Model file for the job. Use its own axes, mm. Face numbers are marked on the shaded views. A direction names the side the tool comes from. Round coordinates to 2 decimals unless told otherwise and drop trailing zeros. Loops run counter-clockwise (first coordinate to the right, second up) from the corner with the lowest first, then second, coordinate; pieces in that order, holes last.
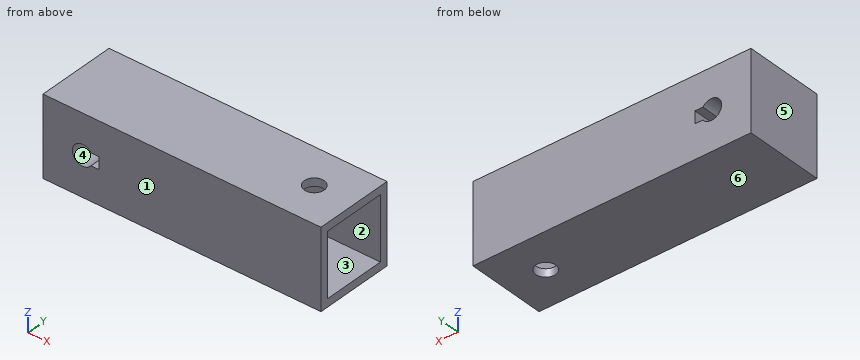
from build123d import *

# Parameters (mm, degrees)
SKETCH2_W               = 140
SKETCH2_H               = 40
SKETCH2_R               = 5.2
BOSS_EXTRUDE1_DEPTH     = 40
CUT_EXTRUDE1_DEPTH      = 84.066238629
CUT_EXTRUDE1_DEPTH_BACK = 84.066238629
SKETCH3_R               = 5
CUT_EXTRUDE5_DEPTH      = 84.066238629
CUT_EXTRUDE5_DEPTH_BACK = 84.066238629
SKETCH7_W               = 2
SKETCH7_H               = 6.131883886
CUT_EXTRUDE6_START      = 70
SKETCH8_W               = 32
SKETCH8_H               = 32
CUT_EXTRUDE6_DEPTH      = 80


with BuildPart() as part:
    # Sketch2 → Boss-Extrude1 (new body)
    with BuildSketch(Plane(origin=(0, 0, 0), x_dir=(1, 0, 0), z_dir=(0, 1, 0))):
        Rectangle(SKETCH2_W, SKETCH2_H)
        with Locations(Location((-50, 0, 0), (0, 0, 270))):
            Circle(SKETCH2_R, mode=Mode.SUBTRACT)
    extrude(amount=BOSS_EXTRUDE1_DEPTH)

    # Sketch3 → Cut-Extrude1 (cut, two sides: drawn at the far end of the back side and taken through both)
    with BuildSketch(Plane.XY.offset(-CUT_EXTRUDE1_DEPTH_BACK)):
        with Locations((50, 20)):
            Circle(SKETCH3_R)
    extrude(amount=CUT_EXTRUDE1_DEPTH + CUT_EXTRUDE1_DEPTH_BACK, mode=Mode.SUBTRACT)

    # Sketch7 → Cut-Extrude5 (cut, two sides: drawn at the far end of the back side and taken through both)
    with BuildSketch(Plane(origin=(0, 0, 0), x_dir=(1, 0, 0), z_dir=(0, 1, 0)).offset(-CUT_EXTRUDE5_DEPTH_BACK)):
        with Locations((-42.8, 0)):
            Rectangle(SKETCH7_W, SKETCH7_H)
        with Locations((-44.8, 0)):
            Rectangle(SKETCH7_W, SKETCH7_H)
    extrude(amount=CUT_EXTRUDE5_DEPTH + CUT_EXTRUDE5_DEPTH_BACK, mode=Mode.SUBTRACT)

    # Sketch8 → Cut-Extrude6 (cut)
    with BuildSketch(Plane(origin=(0, 0, 0), x_dir=(0, 0, -1), z_dir=(1, 0, 0)).offset(CUT_EXTRUDE6_START)):
        with Locations((0, 20)):
            Rectangle(SKETCH8_W, SKETCH8_H)
    extrude(amount=-CUT_EXTRUDE6_DEPTH, mode=Mode.SUBTRACT)


solid = part.part
Q1. Slice it at B-B on y = 20. Give the cut face in (x, z), plus the area to 3 significant figures.
Q2. Slice it at A-A on x = -50. Give the cut face in (y, z), plus the area to 3 significant figures.
Q3. Pull direction Z, two halves, no side cores. Call the marked faces 3, 4, 5 and 6: pulls with the +Z half, pulls with the -Z half, needs draft (parallel to the pull), parting line crosses it, or undercut.
Q4. Flat gauge pin, fed straight in: P1, Ø2, axis at y = 10, z = -11, coming from the +X side. Where does the tip first touch, or does it go through?
Q5. Slice it at C-C on z = 1. Give the cut face in (x, y), plus the area to 3 significant figures.
Q6. Slice it at D-D on y = 34. Give the cut face in (x, z).
Q7. Tool access for the marked faces 1 and 2: list every direction of +Z, -Z, +X, -X, +Y, -Y with a clear straight run to the whole face (end or side of a thin tool).
Q8. Probe line 1 (X direction, y = 20, z = 17.55); line 2 (Y direction, x = 35, z = 7); line 3 (Z direction, x = 27, y = 32.5). List the from-to ranges inside material, lowest first.
Reply:
1. outline: (-70, -20) - (45, -20) - (45, -16) - (-10, -16) - (-10, 16) - (45, 16) - (45, 20) - (-70, 20) - close; (55, -20) - (70, -20) - (70, -16) - (55, -16) - close; (55, 16) - (70, 16) - (70, 20) - (55, 20) - close; hole (-45.8, -3.07) - (-41.8, -3.07) - (-41.8, 3.07) - (-45.8, 3.07) arc R5.2 ccw (long way) to start
1. area: 2,850 mm2
2. outline: (0, -20) - (40, -20) - (40, -5.2) - (0, -5.2) - close; (0, 5.2) - (40, 5.2) - (40, 20) - (0, 20) - close
2. area: 1,180 mm2
3. face 3: undercut
3. face 4: undercut
3. face 5: needs draft
3. face 6: pulls with the -Z half
4. P1: stops at x = -10
5. outline: (-70, 0) - (-55.1, 0) - (-55.1, 40) - (-70, 40) - close; (-41.8, 0) - (70, 0) - (70, 4) - (-10, 4) - (-10, 36) - (70, 36) - (70, 40) - (-41.8, 40) - close
5. area: 2,510 mm2
6. outline: (-70, -20) - (70, -20) - (70, -16) - (-10, -16) - (-10, 16) - (70, 16) - (70, 20) - (-70, 20) - close; hole (-45.8, -3.07) - (-41.8, -3.07) - (-41.8, 3.07) - (-45.8, 3.07) arc R5.2 ccw (long way) to start
7. face 1: +Z, -Z, +X, -X, -Y
7. face 2: +X
8. line 1: x = -70 to 45, 55 to 70
8. line 2: y = 0 to 4, 36 to 40
8. line 3: z = -20 to -16, 16 to 20
